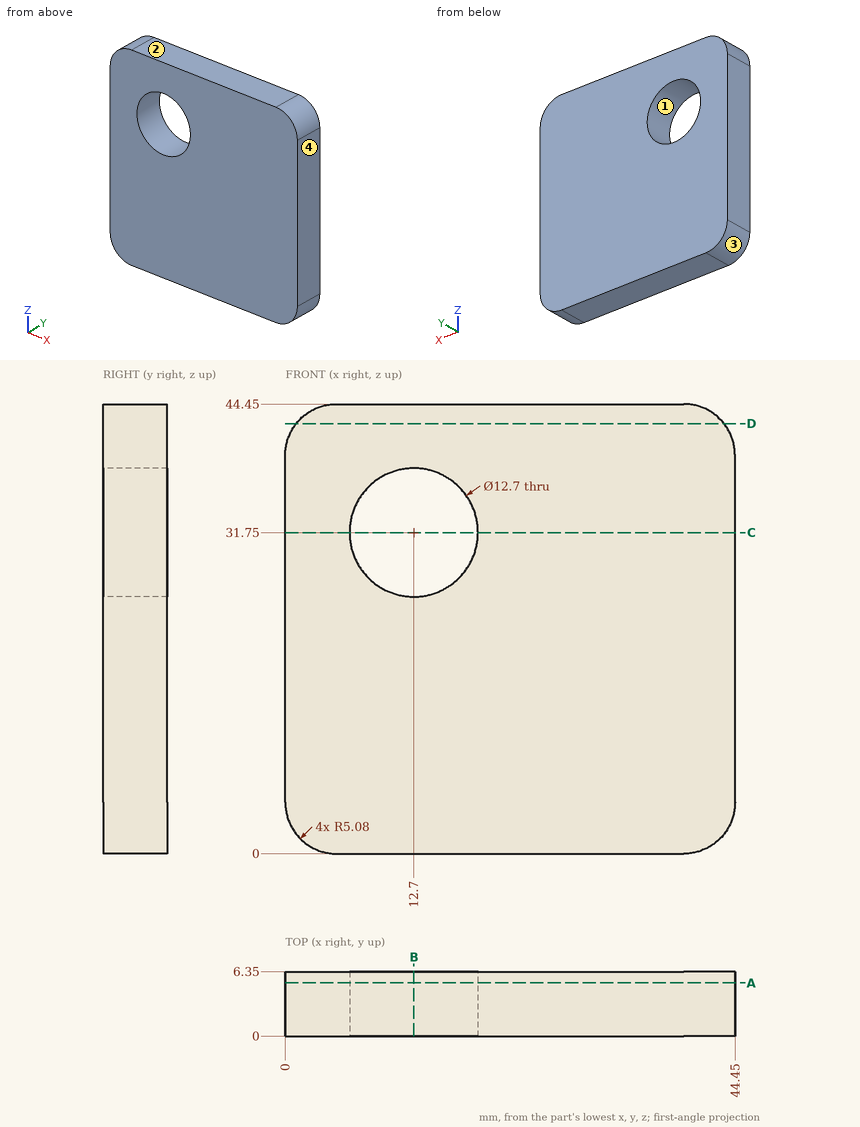
Study the drawing (mm; zero at the part's minimum x, y, z) and answer. Give positions to 0.01 mm unless a question says otherwise; leave off trailing zeros. Order: outer loops, then holes, each group sorted by start corner. A loop starts at its lowest first (then second) coordinate and runs counter-clockwise, first axis right, second up.
1. Section B-B, the plane x = 12.7 is taken. Determine the outline of the cut face in (y, z), and give its area (3 significant figures).
Result sheet:
outline: (0, 0) - (6.35, 0) - (6.35, 25.4) - (0, 25.4) - close; (0, 38.1) - (6.35, 38.1) - (6.35, 44.45) - (0, 44.45) - close
area: 202 mm2
2. Section A-A, the plane y = 5.25 is taken. Determine the outline of the cut face in (x, z).
Result sheet:
outline: (0, 5.08) arc R5.08 ccw to (5.08, 0) - (39.37, 0) arc R5.08 ccw to (44.45, 5.08) - (44.45, 39.37) arc R5.08 ccw to (39.37, 44.45) - (5.08, 44.45) arc R5.08 ccw to (0, 39.37) - close; hole circle Ø12.7 at (12.7, 31.75)
3. Section C-C, the plane z = 31.75 is taken. Determine the outline of the cut face in (x, y), and give its area (3 significant figures).
Result sheet:
outline: (0, 0) - (6.35, 0) - (6.35, 6.35) - (0, 6.35) - close; (19.05, 0) - (44.45, 0) - (44.45, 6.35) - (19.05, 6.35) - close
area: 202 mm2
4. This flat-tipped pin is pushed along its axis until it touches: P1, Ø3, axis at x = 19.5, z = 28.5, coming from the -Y side. Where does it stop, or does it pass through?
Result sheet:
P1: stops at y = 0
5. The mould has two halves that part along X. Classify the marked faces 1, 2, 3 and 4: released by +X, released by -X, zero draft, split by the parting line, or undercut.
Result sheet:
face 1: undercut
face 2: zero draft
face 3: released by -X
face 4: released by +X
6. Straight lines are drawn through the part: L1, parallel to Z at x = 12.7, y = 4.75; L2, parallel to X at y = 5.75, z = 33.5; L3, parallel to Z at x = 15, y = 5.5. For each, find the intervals that lie inside material, in ascending order.
Result sheet:
L1: z = 0 to 25.4, 38.1 to 44.45
L2: x = 0 to 6.6, 18.8 to 44.45
L3: z = 0 to 25.83, 37.67 to 44.45
7. Section D-D, the plane z = 42.5 is taken. Determine the outline of the cut face in (x, y).
Result sheet:
outline: (1.08, 0) - (43.37, 0) - (43.37, 6.35) - (1.08, 6.35) - close
